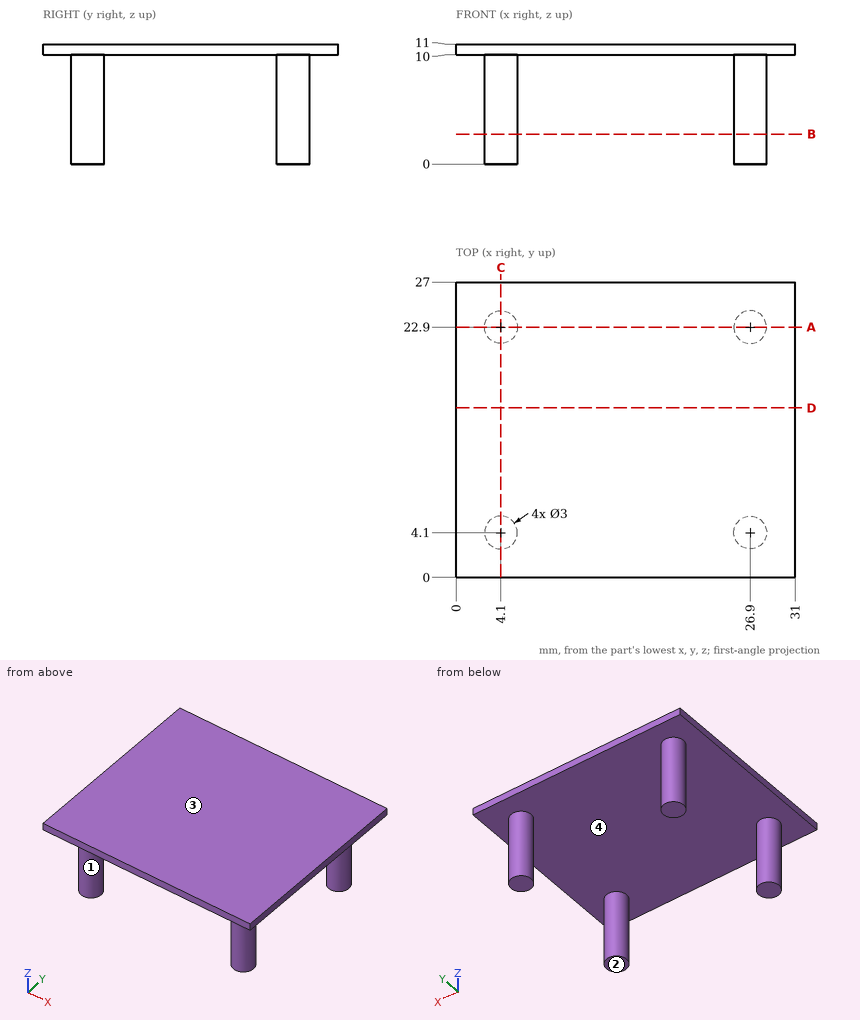
Verification items for this drawing (mm, ordinates from the low corner). A direction names the side the tool comes from. Coordinates: 2 decimals unless noted, no trailing zeros. Loops run counter-clockwise (first coordinate to the right, second up) from the corner with the lowest first, then second, coordinate; pieces in that order, holes last. Notation, with made-up numbers: (52.5, 70.25) -> (85.5, 70.25) arc R13 cw to (85.5, 85.25) -> close; hole circle Ø3 at (1.25, 46.5). An arc over 180 degrees is marked (long way). Put each result on its own line as item: value.
1. Thickness scan on line 1 (Z direction, x = 29, y = 1); line 2 (X direction, y = 5, z = 1); line 3 (Y direction, x = 3, z = 7). Record the ranges inside material, lowest first.
Result set:
line 1: z = 10 to 11
line 2: x = 2.9 to 5.3, 25.7 to 28.1
line 3: y = 3.08 to 5.12, 21.88 to 23.92
2. Section check C-C, the plane x = 4.1. Record the boundary of the cut face in (y, z), then the cut area to 3 significant figures.
Result set:
outline: (0, 10) -> (2.6, 10) -> (2.6, 0) -> (5.6, 0) -> (5.6, 10) -> (21.4, 10) -> (21.4, 0) -> (24.4, 0) -> (24.4, 10) -> (27, 10) -> (27, 11) -> (0, 11) -> close
area: 87.0 mm^2
3. Mould release check, pull along X, two halves, no side actions. Record for the marked faces 3 and 4: pulls with the +X half, pulls with the -X half, needs draft (parallel to the pull), parting line crosses it, or undercut.
Result set:
face 3: needs draft
face 4: undercut
4. Section check D-D, the plane y = 15.5. Record the boundary of the cut face in (x, z).
Result set:
outline: (0, 10) -> (31, 10) -> (31, 11) -> (0, 11) -> close
5. Gauge pin test, flat end, axial feed: P1, Ø10, axis at x = 13, y = 13.5, coming from the -Z side. Record the tip position at first contact, or that the pin passes through.
Result set:
P1: stops at z = 10
6. Section check B-B, the plane z = 2.75. Record the boundary of the cut face in (x, y).
Result set:
outline: circle Ø3 at (4.1, 4.1); circle Ø3 at (4.1, 22.9); circle Ø3 at (26.9, 4.1); circle Ø3 at (26.9, 22.9)
7. Tool access check on the marked faces 1 and 2. Record the directions out of +Z, -Z, +X, -X, +Y, -Y that give a thin tool (end or side, any length) a straight path to the whole face; none if there is none.
Result set:
face 1: -Z
face 2: -Z, +X, -X, +Y, -Y
8. Section check A-A, the plane y = 22.9. Record the boundary of the cut face in (x, z).
Result set:
outline: (0, 10) -> (2.6, 10) -> (2.6, 0) -> (5.6, 0) -> (5.6, 10) -> (25.4, 10) -> (25.4, 0) -> (28.4, 0) -> (28.4, 10) -> (31, 10) -> (31, 11) -> (0, 11) -> close
